Verification items for the finished model (mm, model axes). Coordinates: 2 decimals unless noted, no trailing zeros. Order: outer loops, then holes, each group sorted by start corner. A loop starts at its lowest first (then second) coordinate and runs counter-clockwise, first axis right, second up. Notation, with made-up numbers: M -15,-20 L 17,-20 A36 cw 17,17 Z; hole C 40,35.25 d8. An arc over 180 degrees is marked long. Return JSON: item names as keys, results as strings. Group by question number.
1. Section check D-D, the plane z = 7.25. Record the cut outline in (x, y), plus the area to 3 significant figures.
2. Section check A-A, the plane x = 4. Record the cut outline in (y, z), plus the area to 3 significant figures.
3. Mould release check, pull along Z, two halves, no side actions. Record for faces 1 (the flat face through (0, 0, 4.05)), 2 (the flat face through (6.75, 0, 7)), 3 (the flat face through (16.825, 0, 7)): +Z half, -Z half, draft (parallel to the pull), parting line (faces both ways), or undercut.
4. Section check B-B, the plane z = 10.25. Record the cut outline in (x, y), plus the area to 3 significant figures.
5. Section check C-C, the plane x = 8.5. Record the cut outline in (y, z), plus the area to 3 significant figures.
6. Gauge pin test, flat end, axial feed: pin 1 (1 mm diameter, centred on x = 12, y = -2, fed in from +Z). Record the tip position at first contact, or that the pin passes through.
7. Material ranges on line 1 along Z through (x, y) = (3, 0.25); line 2 along Y through (x, z) = (13, 8.25); line 3 along X through (y, z) = (2.75, 4.5), recorded low to high.
```python
from build123d import *

# Parameters (mm, degrees)
BOSS_EXTRUDE1_DEPTH = 13.5
SKETCH2_W           = 5.4
SKETCH2_H           = 14
CUT_EXTRUDE1_DEPTH  = 13.5
SKETCH3_R           = 12.152813435
SKETCH3_R_2         = 8
CUT_EXTRUDE2_DEPTH  = 24.574911634
BOSS_EXTRUDE2_DEPTH = 32.5
CUT_EXTRUDE4_DEPTH  = 25.746559571
SKETCH8_W           = 15.715396091
SKETCH8_H           = 5.4
CUT_EXTRUDE5_DEPTH  = 23.5


with BuildPart() as part:
    # Sketch1 → Boss-Extrude1 (new body)
    with BuildSketch(Plane.XY):
        with BuildLine():
            Line((-6.75, 0.697518811), (-6.75, -0.720756429))
            ThreePointArc((-6.75, -0.720756429), (-5.635274328, -3.766828408), (-3.219489146, -5.931349089))
            Line((-3.219489146, -5.931349089), (16.824911634, -5.931349089))
            Line((16.824911634, -5.931349089), (16.824911634, 5.931349089))
            Line((16.824911634, 5.931349089), (-3.175088366, 5.931349089))
            ThreePointArc((-3.175088366, 5.931349089), (-5.621180267, 3.764308263), (-6.75, 0.697518811))
        make_face()
    extrude(amount=BOSS_EXTRUDE1_DEPTH)

    # Sketch2 → Cut-Extrude1 (cut)
    with BuildSketch(Plane.ZY.offset(6.75)):
        with Locations((6.75, 0)):
            Rectangle(SKETCH2_W, SKETCH2_H)
    extrude(amount=-CUT_EXTRUDE1_DEPTH, mode=Mode.SUBTRACT)

    # Sketch3 → Cut-Extrude2 (cut, through all)
    with BuildSketch(Plane(origin=(16.824911634, 0, 0), x_dir=(0, 0, -1), z_dir=(1, 0, 0))):
        with Locations((-6.746559471, 0)):
            Circle(SKETCH3_R)
        with Locations((-6.746559471, 0)):
            Circle(SKETCH3_R_2, mode=Mode.SUBTRACT)
    extrude(amount=-CUT_EXTRUDE2_DEPTH, mode=Mode.SUBTRACT)

    # Sketch4 → Boss-Extrude2 (add)
    with BuildSketch(Plane(origin=(16.824911634, 0, 0), x_dir=(0, 0, -1), z_dir=(1, 0, 0))):
        with BuildLine():
            Line((-1.37821727, -5.931349089), (-12.114901672, -5.931349089))
            ThreePointArc((-12.114901672, -5.931349089), (-6.746559471, -8), (-1.37821727, -5.931349089))
        make_face()
        with BuildLine():
            Line((-13.5, -4.288477704), (-13.5, 4.288477704))
            ThreePointArc((-13.5, 4.288477704), (-14.746559471, 0), (-13.5, -4.288477704))
        make_face()
        with BuildLine():
            ThreePointArc((-1.37821727, 5.931349089), (-6.746559471, 8), (-12.114901672, 5.931349089))
            Line((-12.114901672, 5.931349089), (-1.37821727, 5.931349089))
        make_face()
        with BuildLine():
            ThreePointArc((1.253440529, 0), (0.933690387, 2.239143166), (0, 4.299294745))
            Line((0, 4.299294745), (0, -4.299294745))
            ThreePointArc((0, -4.299294745), (0.933690387, -2.239143166), (1.253440529, 0))
        make_face()
    extrude(amount=-BOSS_EXTRUDE2_DEPTH)

    # Sketch7 → Cut-Extrude4 (cut, through all)
    with BuildSketch(Plane.XY.offset(-10)):
        with BuildLine():
            Line((-6.656945588, -0.70913762), (-6.656945588, 0.70913762))
            ThreePointArc((-6.656945588, 0.70913762), (-6.164537152, 2.610801109), (-5.141365169, 4.287675936))
            ThreePointArc((-5.141365169, 4.287675936), (-4.213671695, 5.202189114), (-3.126434734, 5.91973028))
            ThreePointArc((-3.126434734, 5.91973028), (-1.594815167, 6.522683652), (0.037211277, 6.736928732))
            Line((0.037211277, 6.736928732), (17.631347577, 6.736928732))
            Line((17.631347577, 6.736928732), (17.631347577, 9.936708938))
            Line((17.631347577, 9.936708938), (-17.152869805, 9.936708938))
            Line((-17.152869805, 9.936708938), (-17.769305726, -9.133185925))
            Line((-17.769305726, -9.133185925), (18.753818668, -9.133185925))
            Line((18.753818668, -9.133185925), (18.753818668, -6.692966124))
            Line((18.753818668, -6.692966124), (0.148341476, -6.692966124))
            ThreePointArc((0.148341476, -6.692966124), (-1.514021871, -6.521160825), (-3.082033954, -5.942967898))
            ThreePointArc((-3.082033954, -5.942967898), (-4.182346183, -5.227406732), (-5.121896627, -4.310913554))
            ThreePointArc((-5.121896627, -4.310913554), (-6.158610107, -2.62475185), (-6.656945588, -0.70913762))
        make_face()
    extrude(amount=CUT_EXTRUDE4_DEPTH, mode=Mode.SUBTRACT)

    # Sketch8 → Cut-Extrude5 (cut)
    with BuildSketch(Plane.XZ.offset(6.692966124)):
        with Locations((-1.107698046, 6.75)):
            Rectangle(SKETCH8_W, SKETCH8_H)
    extrude(amount=-CUT_EXTRUDE5_DEPTH, mode=Mode.SUBTRACT)


solid = part.part
```
Answers follow:
{
 "1": {"outline": "M -0.15,-6.69 A6.69 ccw 0.15,-6.69 Z; M 6.75,-6.69 L 16.82,-6.69 L 16.82,6.74 L 6.75,6.74 Z", "area": "135 mm^2"},
 "2": {"outline": "M -6.69,2.36 A8 ccw 6.74,2.43 L 6.74,4.05 L -6.69,4.05 Z; M -6.69,9.45 L 6.74,9.45 L 6.74,11.06 A8 ccw -6.69,11.13 Z", "area": "113 mm^2"},
 "3": {"face 1": "undercut", "face 2": "undercut", "face 3": "draft"},
 "4": {"outline": "M -6.66,-0.71 A6.69 ccw 0.15,-6.69 L 16.82,-6.69 L 16.82,6.74 L 0.04,6.74 A6.75 ccw -3.13,5.92 A6.69 ccw -6.66,0.71 Z", "area": "296 mm^2"},
 "5": {"outline": "M -6.69,2.36 A8 ccw 6.74,2.43 L 6.74,11.06 A8 ccw -6.69,11.13 Z", "area": "186 mm^2"},
 "6": {"pin 1": "z = 14.6"},
 "7": {"line 1": "-1.25 to 4.05, 9.45 to 14.74", "line 2": "-6.69 to 6.74", "line 3": "6.75 to 16.82"}
}
